```python
from build123d import *

# Parameters (mm, degrees)
ESQUISSE2_W                  = 215.9
ESQUISSE2_H                  = 152.4
BOSS_EXTRU_1_DEPTH           = 6.35
ENL_V_MAT_EXTRU_1_DEPTH      = 133.287433266
ENL_V_MAT_EXTRU_1_DEPTH_BACK = 133.287433266
ESQUISSE3_W                  = 12.7
ESQUISSE3_H                  = 6.35
CONG_1_R                     = 12.7
ENL_V_MAT_EXTRU_2_DEPTH      = 133.287433266


with BuildPart() as part:
    # Esquisse2 → Boss.-Extru.1 (new body)
    with BuildSketch(Plane(origin=(0, 0, 0), x_dir=(1, 0, 0), z_dir=(0, 1, 0))):
        Rectangle(ESQUISSE2_W, ESQUISSE2_H)
    extrude(amount=BOSS_EXTRU_1_DEPTH)

    # Esquisse3 → Enlèv. mat.-Extru.1 (cut, two sides: drawn at the far end of the back side and taken through both)
    with BuildSketch(Plane(origin=(0, 6.35, 0), x_dir=(1, 0, 0), z_dir=(0, 1, 0)).offset(-ENL_V_MAT_EXTRU_1_DEPTH_BACK)):
        with Locations((-88.9, 73.025)):
            Rectangle(ESQUISSE3_W, ESQUISSE3_H)
        with Locations((-88.9, 53.975)):
            Rectangle(ESQUISSE3_W, ESQUISSE3_H)
        with Locations((88.9, 53.975)):
            Rectangle(ESQUISSE3_W, ESQUISSE3_H)
        with Locations((88.9, 73.025)):
            Rectangle(ESQUISSE3_W, ESQUISSE3_H)
    extrude(amount=ENL_V_MAT_EXTRU_1_DEPTH + ENL_V_MAT_EXTRU_1_DEPTH_BACK, mode=Mode.SUBTRACT)

    # Congé1
    cong_1_edges = [part.edges().sort_by_distance(p)[0] for p in [
        (107.95, 3.175, 76.2),
        (-107.95, 3.175, 76.2),
    ]]
    fillet(cong_1_edges, radius=CONG_1_R)

    # Esquisse4 → Enlèv. mat.-Extru.2 (cut, through all)
    with BuildSketch(Plane(origin=(0, 6.35, 0), x_dir=(1, 0, 0), z_dir=(0, 1, 0))):
        with BuildLine():
            Line((-44.45, 38.1), (44.45, 38.1))
            ThreePointArc((44.45, 38.1), (48.940128061, 36.240128061), (50.8, 31.75))
            Line((50.8, 31.75), (50.8, -57.15))
            ThreePointArc((50.8, -57.15), (48.940128061, -61.640128061), (44.45, -63.5))
            Line((44.45, -63.5), (-44.45, -63.5))
            ThreePointArc((-44.45, -63.5), (-48.940128061, -61.640128061), (-50.8, -57.15))
            Line((-50.8, -57.15), (-50.8, 31.75))
            ThreePointArc((-50.8, 31.75), (-48.940128061, 36.240128061), (-44.45, 38.1))
        make_face()
    extrude(amount=-ENL_V_MAT_EXTRU_2_DEPTH, mode=Mode.SUBTRACT)


solid = part.part
```
Check sheet for the modelled part. Datum: model origin and axes. Units: mm. A direction names the side the tool comes from. Round coordinates to 2 decimals unless told otherwise and drop trailing zeros. Loops run counter-clockwise (first coordinate to the right, second up) from the corner with the lowest first, then second, coordinate; pieces in that order, holes last. Notation, with made-up numbers: (56.5, 61) - (72.5, 61) arc R35 cw to (72.5, 97) - close; hole circle Ø4 at (65.25, 63.5). An arc over 180 degrees is marked (long way). Answer as a JSON object with one key per item and string values. Group by question number.
Q1. Gauge pin test, flat end, axial feed: P1, Ø1.9, axis at x = 90.5, y = 4, coming from the -Z side. Record the tip position at first contact, or that the pin passes through.
Q2. Sectioned sample at B-B, the plane x = -33. Enter the section's corners in (y, z).
Q3. Set-up check for faces 1 (the face through (-89, 3, -69.85)), 2 (the face through (104.13, 3.22, 72.58)), 3 (the face through (-50.8, 3, 13)): record each of +Z, -Z, +X, -X, +Y, -Y from which the full face is reachable in a straight line by a thin tool's end or side.
Q4. Mould release check, pull along Z, two halves, no side actions. Record for faces 4 (the face through (-1, 3, -76.2)), 5 (the face through (82.55, 3, -73)), 6 (the face through (89, 3, -50.8)): released by +Z, released by -Z, zero draft, split by the parting line, or undercut.
Q5. Scan lines: line 1 along X through (y, z) = (2.25, -53.5); line 2 along X through (y, z) = (3.5, -24); line 3 along Z through (x, y) = (17.5, 5.5). Record each from-to range of solid material in increasing order. Write a range as [from, to].
Q6. Sectioned sample at C-C, the plane y = 1. Count the separate pieces of the cut face and the enclosed holes in it, plus the area to 3 significant figures.
Q7. Sectioned sample at D-D, the plane z = -12. Enter the section's corners in (x, y).
Q8. Sectioned sample at A-A, the plane z = -55. Enter the section's corners in (x, y).
Solution:
{
 "1": {"P1": "stops at z = -69.85"},
 "2": {"outline": "(0, -76.2) - (6.35, -76.2) - (6.35, -38.1) - (0, -38.1) - close; (0, 63.5) - (6.35, 63.5) - (6.35, 76.2) - (0, 76.2) - close"},
 "3": {"face 1": "-Z, +Y, -Y", "face 2": "+Z, +X, +Y, -Y", "face 3": "+Y, -Y"},
 "4": {"face 4": "released by -Z", "face 5": "zero draft", "face 6": "undercut"},
 "5": {"line 1": "x = [-107.95, -95.25], [-82.55, 82.55], [95.25, 107.95]", "line 2": "x = [-107.95, -50.8], [50.8, 107.95]", "line 3": "z = [-76.2, -38.1], [63.5, 76.2]"},
 "6": {"separate pieces": "1", "enclosed holes": "3", "area": "22,200 mm²"},
 "7": {"outline": "(-107.95, 0) - (-50.8, 0) - (-50.8, 6.35) - (-107.95, 6.35) - close; (50.8, 0) - (107.95, 0) - (107.95, 6.35) - (50.8, 6.35) - close"},
 "8": {"outline": "(-107.95, 0) - (-95.25, 0) - (-95.25, 6.35) - (-107.95, 6.35) - close; (-82.55, 0) - (82.55, 0) - (82.55, 6.35) - (-82.55, 6.35) - close; (95.25, 0) - (107.95, 0) - (107.95, 6.35) - (95.25, 6.35) - close"}
}
